The model under review builds one solid part; all positions refer to its coordinate system, in mm. A direction names the side the tool comes from. Coordinates: 2 decimals unless noted, no trailing zeros. Write each loop counter-clockwise with the first axis right and the second up, starting at its lowest first coordinate (ties: lowest second). Pieces come first, ordered by that corner, then holes.
```python
from build123d import *

# Parameters (mm, degrees)
F0_R     = 30.1625
F0_R_2   = 26.9875
F1_DEPTH = 3.96875
F2_R     = 36.329519
F2_R_2   = 28.575
F3_DEPTH = 2.2225
F4_W     = 25.4
F4_H     = 40.857697
F5_DEPTH = 12.7


with BuildPart() as f1:
    # F0 (on Top) → F1 (new body, symmetric)
    with BuildSketch(Plane.XY):
        Circle(F0_R)
        Circle(F0_R_2, mode=Mode.SUBTRACT)
    extrude(amount=F1_DEPTH, both=True)

    # F2 (on Top) → F3 (cut, symmetric)
    with BuildSketch(Plane.XY):
        Circle(F2_R)
        Circle(F2_R_2, mode=Mode.SUBTRACT)
    extrude(amount=F3_DEPTH, both=True, mode=Mode.SUBTRACT)

    # F4 (on Top) → F5 (cut, symmetric)
    with BuildSketch(Plane.XY):
        with Locations((0, -20.428848)):
            Rectangle(F4_W, F4_H)
    extrude(amount=F5_DEPTH, both=True, mode=Mode.SUBTRACT)


solid = f1.part
```
Item 1: To check wall thickness, follow line 1 along X through (y, z) = (0, 1.75) (1 decimal); line 2 along X through (y, z) = (-17.5, 0); line 3 along Y through (x, z) = (-0.5, -1.5). State the ranges of each line that lie inside material, in increasing order.
Solved:
line 1: x = -28.6 to -27, 27 to 28.6
line 2: x = -22.59 to -20.54, 20.54 to 22.59
line 3: y = 26.98 to 28.57
Item 2: Take a section at D-D, the plane z = 3.25. Write out the cut boundary in (x, y) (1 decimal).
Solved:
outline: (-12.7, -27.4) - (-12.7, -23.8) arc R27 cw (long way) to (12.7, -23.8) - (12.7, -27.4) arc R30.2 ccw (long way) to start
Item 3: Take a section at B-B, the plane x = 20. Write out the cut boundary in (y, z), plus the area to 3 significant figures.
Solved:
outline: (-22.58, -3.97) - (-18.12, -3.97) - (-18.12, 3.97) - (-22.58, 3.97) - (-22.58, 2.22) - (-20.41, 2.22) - (-20.41, -2.22) - (-22.58, -2.22) - close; (18.12, -3.97) - (22.58, -3.97) - (22.58, -2.22) - (20.41, -2.22) - (20.41, 2.22) - (22.58, 2.22) - (22.58, 3.97) - (18.12, 3.97) - close
area: 51.5 mm2
Item 4: Take a section at A-A, the plane y = 0. Write out the cut boundary in (x, z) (1 decimal).
Solved:
outline: (-30.2, -4) - (-27, -4) - (-27, 4) - (-30.2, 4) - (-30.2, 2.2) - (-28.6, 2.2) - (-28.6, -2.2) - (-30.2, -2.2) - close; (27, -4) - (30.2, -4) - (30.2, -2.2) - (28.6, -2.2) - (28.6, 2.2) - (30.2, 2.2) - (30.2, 4) - (27, 4) - close
Item 5: Take a section at C-C, the plane x = 0. Write out the cut boundary in (y, z) (1 decimal), plus the area to 3 significant figures.
Solved:
outline: (27, -4) - (30.2, -4) - (30.2, -2.2) - (28.6, -2.2) - (28.6, 2.2) - (30.2, 2.2) - (30.2, 4) - (27, 4) - close
area: 18.1 mm2
Item 6: For pin 1 (1 mm diameter, centred on x = -17.5, z = 2.5, fed in from -Y); pin 2 (3 mm diameter, centred on y = -26.5, z = 0, fed in from +X); pin 3 (3 mm diameter, centred on x = 22, y = 23, fed in from -Z); pin 4 (1.8 mm diameter, centred on y = -25.5, z = 0, fed in from -X), all flat-tipped, find the tip position at first contact; note any pin that passes through.
Solved:
pin 1: stops at y = -24.92
pin 2: stops at x = 13.84
pin 3: passes through
pin 4: stops at x = -14.54
Item 7: Mouldability with a two-part tool opening along Y and no side actions: class faces 1 (the face through (1, 26.97, -0.06)), 2 (the face through (1.14, 30.14, -3.08)), 3 (the face through (-12.7, -25, 0)) as pulls with the +Y half, pulls with the -Y half, needs draft (parallel to the pull), parting line crosses it, or undercut.
Solved:
face 1: undercut
face 2: parting line crosses it
face 3: needs draft
Item 8: Machinability: for faces 4 (the face through (12.7, -25, 0)), 5 (the face through (-2.4, 27.1, 3.969)), 6 (the face through (0, 29, -2.222)), which of the approach directions +Z, -Z, +X, -X, +Y, -Y give a long, thin tool a straight path to every point of the face, cutting with its end or side? Answer none if there is none.
Solved:
face 4: +Z, -Z, -Y
face 5: +Z, +X, -X, +Y, -Y
face 6: none
